For this review, take the finished solid that the model builds, in its own axes (mm). Face numbers are marked on the shaded views. A direction names the side the tool comes from. Round coordinates to 2 decimals unless told otherwise and drop trailing zeros. Write each loop counter-clockwise with the first axis right and the second up, starting at its lowest first coordinate (ties: lowest second). Pieces come first, ordered by that corner, then holes. Notation, with made-up numbers: (-36.5, 66.5) -> (15.5, 66.5) arc R17 cw to (15.5, 95.5) -> close; hole circle Ø4 at (55, 56). An arc over 180 degrees is marked (long way). Answer in a Markdown table with one row per item. Add a question column.
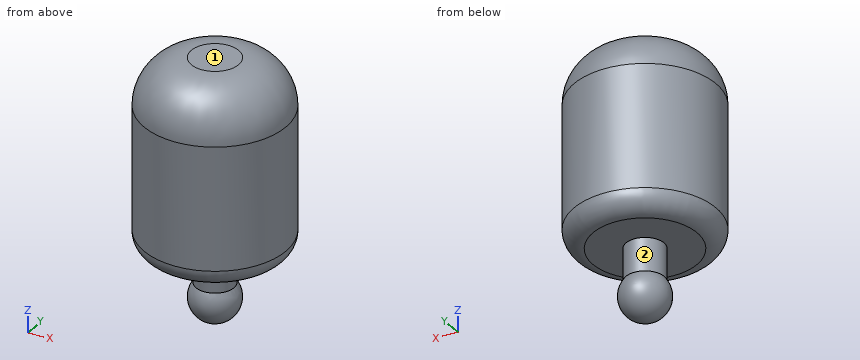
```python
from build123d import *

# Parameters (mm, degrees)
F0_R     = 7.5
F1_DEPTH = 20
F2_R     = 5
F3_R     = 2
F4_DEPTH = 5
F7_R     = 2


with BuildPart() as f1:
    # F0 (on Top) → F1 (new body)
    with BuildSketch(Plane.XY):
        Circle(F0_R)
    extrude(amount=F1_DEPTH)

    # F2
    f2_edges = [f1.edges().sort_by_distance(p)[0] for p in [
        (-7.5, 0, 20),
    ]]
    fillet(f2_edges, radius=F2_R)

    # F3 (on face) → F4 (join)
    with BuildSketch(Plane(origin=(0, 0, 0), x_dir=(1, 0, 0), z_dir=(0, 0, -1))):
        Circle(F3_R)
    extrude(amount=F4_DEPTH)

    # F5 (on face) → F6 (revolve)
    with BuildSketch(Plane(origin=(0, 0, -5), x_dir=(1, 0, 0), z_dir=(0, 0, -1))):
        with BuildLine():
            Line((0, 2), (0, 2.5))
            ThreePointArc((0, 2.5), (-2.5, 0), (0, -2.5))
            Line((0, -2.5), (0, -2))
            ThreePointArc((0, -2), (-2, 0), (0, 2))
        make_face()
        with BuildLine():
            Line((0, -2), (0, 2))
            ThreePointArc((0, 2), (-2, 0), (0, -2))
        make_face()
        with BuildLine():
            ThreePointArc((2, 0), (1.4142135624, 1.4142135624), (0, 2))
            Line((0, 2), (0, -2))
            ThreePointArc((0, -2), (1.4142135624, -1.4142135624), (2, 0))
        make_face()
    revolve(axis=Axis((0, 0, -5), (0, 1, 0)))

    # F7
    f7_edges = [f1.edges().sort_by_distance(p)[0] for p in [
        (-7.5, 0, 0),
    ]]
    fillet(f7_edges, radius=F7_R)


solid = f1.part
```
1. We need section B-B (z = 1.5). Write out the cut boundary in (x, y), plus the area to 3 significant figures.
2. Tool access review of the marked faces 1 and 2: name each direction out of +Z, -Z, +X, -X, +Y, -Y from which nothing blocks a thin tool from reaching the whole face with its end or side.
3. We need section A-A (z = 11.75). Write out the cut boundary in (x, y).
4. For L1, parallel to Z at x = 0.5, y = -0.75; L2, parallel to Z at x = -0.75, y = 1; L3, parallel to X at y = -0.25, z = 13.5, list the stretches that pass through material, from the lowest coordinate up. Write a range as [from, to].
5. Clearance check with flat-ended pins moving along their axes: pin 1 Ø3 at (x, z) = (5, 0.5) entering from +Y; pin 2 Ø2 at (x, y) = (-4, 2) entering from -Z; pin 3 Ø3 at (x, z) = (3.5, 6) entering from -Y; pin 4 Ø2 at (x, y) = (0, 0.5) entering from -Z. State where each tip first meets the part, or that it passes through.
Response:
| question | item | result |
|---|---|---|
| 1 | outline | circle Ø14.87 at (0, 0) |
| 1 | area | 174 mm2 |
| 2 | face 1 | +Z, +X, -X, +Y, -Y |
| 2 | face 2 | none |
| 3 | outline | circle Ø15 at (0, 0) |
| 4 | L1 | [-7.33, -6.79], [-5, 20] |
| 4 | L2 | [-7.17, -6.56], [-5, 20] |
| 4 | L3 | [-7.5, 7.5] |
| 5 | pin 1 | y = 6.36 |
| 5 | pin 2 | z = 0 |
| 5 | pin 3 | y = -7.23 |
| 5 | pin 4 | z = -7.5 |
